Geometry check sheet. Reference: drawing and pictorial views, mm from the part's lowest x, y, z. A direction names the side the tool comes from. Round coordinates to 2 decimals unless told otherwise and drop trailing zeros. Loops run counter-clockwise (first coordinate to the right, second up) from the corner with the lowest first, then second, coordinate; pieces in that order, holes last. Notation, with made-up numbers: (84, 24.25) -> (143, 24.25) arc R19 cw to (143, 54.25) -> close; hole circle Ø1 at (49, 41). An arc over 180 degrees is marked (long way). Write item = value, one per line.
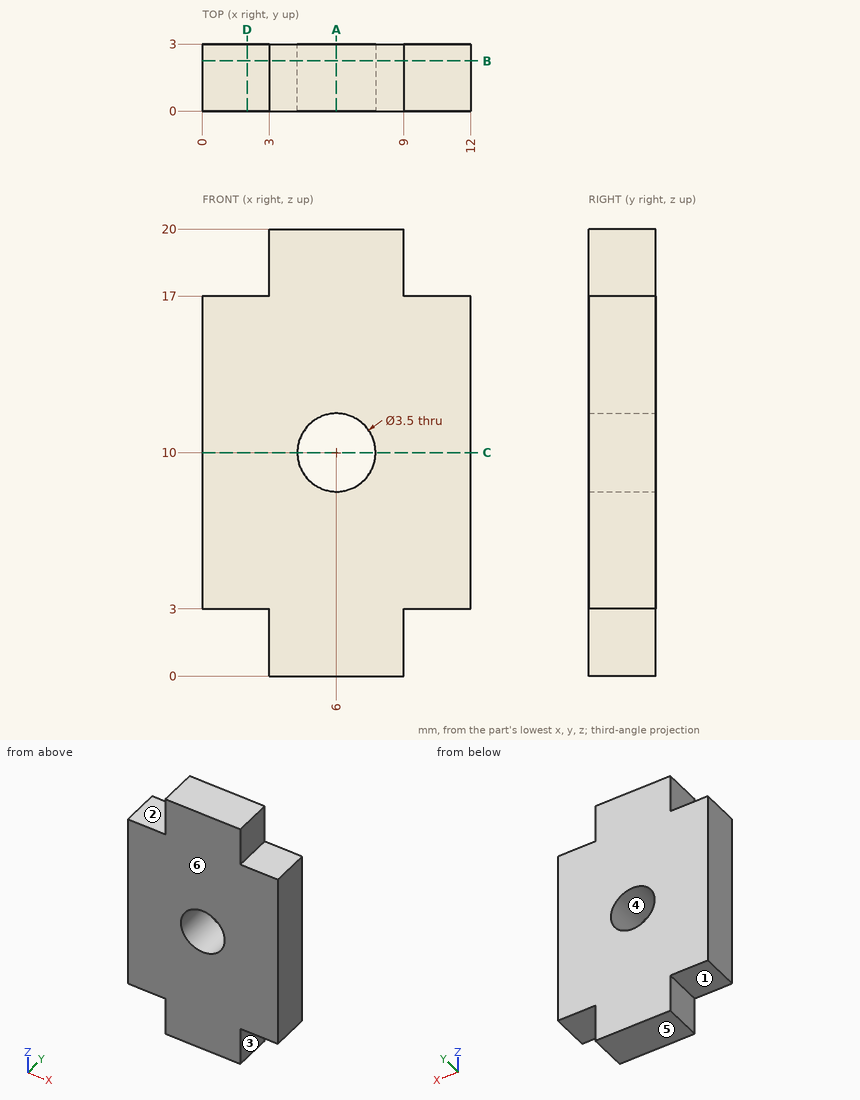
(1) Sectioned sample at C-C, the plane z = 10. Record the cut outline in (x, y).
Filled sheet:
outline = (0, 0) -> (4.25, 0) -> (4.25, 3) -> (0, 3) -> close; (7.75, 0) -> (12, 0) -> (12, 3) -> (7.75, 3) -> close
(2) Material ranges on probe 1 along Z at (x, y) = (6, 2); probe 2 along Z at (x, y) = (5.25, 2.8); probe 3 along X at (y, z) = (2.85, 17.75), recorded low to high. Write a range as from..to.
Filled sheet:
probe_1 = 0..8.25, 11.75..20
probe_2 = 0..8.42, 11.58..20
probe_3 = 3..9
(3) Set-up check for the marked faces 1, 2 and 3: record each of +Z, -Z, +X, -X, +Y, -Y from which the full face is reachable in a straight line by a thin tool's end or side.
Filled sheet:
face_1 = -Z, -X, +Y, -Y
face_2 = +Z, -X, +Y, -Y
face_3 = -Z, +X, +Y, -Y
(4) Sectioned sample at D-D, the plane x = 2. Record the cut outline in (y, z), and give its area (3 significant figures).
Filled sheet:
outline = (0, 3) -> (3, 3) -> (3, 17) -> (0, 17) -> close
area = 42.0 mm2
(5) Draft check along Z on the marked faces 4, 5 and 6. Enter one of: released by +Z, released by -Z, zero draft, split by the parting line, or undercut.
Filled sheet:
face_4 = undercut
face_5 = released by -Z
face_6 = zero draft
(6) Sectioned sample at B-B, the plane y = 2.25. Record the cut outline in (x, z), and give its area (3 significant figures).
Filled sheet:
outline = (0, 3) -> (3, 3) -> (3, 0) -> (9, 0) -> (9, 3) -> (12, 3) -> (12, 17) -> (9, 17) -> (9, 20) -> (3, 20) -> (3, 17) -> (0, 17) -> close; hole circle Ø3.5 at (6, 10)
area = 194 mm2
(7) Go/stop test with flat-tipped pins: pin 1 Ø0.9 at (x, y) = (1, 1) entering from -Z; pin 2 Ø0.9 at (x, y) = (1, 1.5) entering from +Z; pin 3 Ø1.5 at (y, z) = (1.5, 18) entering from -X. Record where each tip stops, or that it passes through.
Filled sheet:
pin_1 = 3
pin_2 = 17
pin_3 = 3
(8) Sectioned sample at A-A, the plane x = 6. Record the cut outline in (y, z).
Filled sheet:
outline = (0, 0) -> (3, 0) -> (3, 8.25) -> (0, 8.25) -> close; (0, 11.75) -> (3, 11.75) -> (3, 20) -> (0, 20) -> close
